from build123d import *

# Parameters (mm, degrees)
F0_W     = 355.6
F0_H     = 355.6
F1_DEPTH = 50.8
F3_DEPTH = 6.35
F4_DEPTH = 6.35


with BuildPart() as f1:
    # F0 (on Front) → F1 (new body)
    with BuildSketch(Plane.XZ):
        Rectangle(F0_W, F0_H)
    extrude(amount=F1_DEPTH)

    # F2 (on face) → F3 (cut)
    with BuildSketch(Plane.XZ.offset(50.8)):
        Polygon((-167.600538, 131.020906), (-171.194881, 122.465245), (101.947516, 55.141423), (104.141387, 64.042271), align=None)
        Polygon((-77.381766, -53.872798), (-73.398896, -66.51783), (163.904211, 8.226743), (162.432873, 21.662845), align=None)
        Polygon((96.553348, -157.102942), (-157.932714, -88.089772), (-160.472856, -99.545852), (93.485428, -168.415896), align=None)
    extrude(amount=-F3_DEPTH, mode=Mode.SUBTRACT)

    # F2 (on face) → F4 (cut)
    with BuildSketch(Plane.XZ.offset(50.8)):
        Polygon((-167.600538, 131.020906), (-171.194881, 122.465245), (101.947516, 55.141423), (104.141387, 64.042271), align=None)
        Polygon((-77.381766, -53.872798), (-73.398896, -66.51783), (163.904211, 8.226743), (162.432873, 21.662845), align=None)
        Polygon((96.553348, -157.102942), (-157.932714, -88.089772), (-160.472856, -99.545852), (93.485428, -168.415896), align=None)
    extrude(amount=-F4_DEPTH, mode=Mode.SUBTRACT)


solid = f1.part
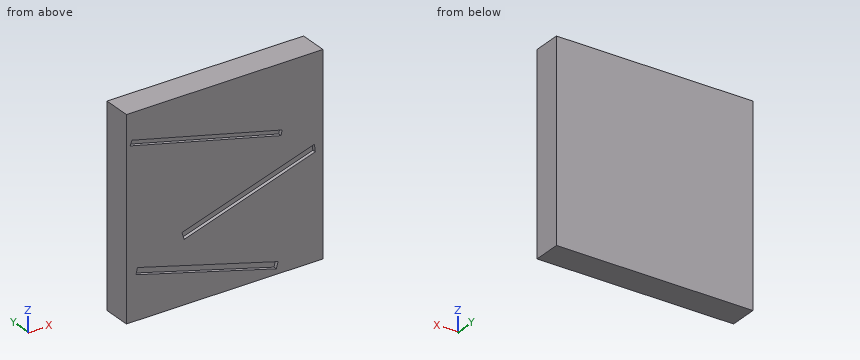
Input: part model. Units: mm. Frame: model coordinates. Give positions to 0.01 mm unless a question says otherwise; leave off trailing zeros. Loops run counter-clockwise (first coordinate to the right, second up) from the corner with the lowest first, then second, coordinate; pieces in that order, holes last. Notation, with made-up numbers: (71, -10) -> (100, -10) arc R28 ccw to (100, 25) -> close; hole circle Ø9 at (-11.75, 27.5). An arc over 180 degrees is marked (long way). Answer as a JSON object with one key per item and string values. Group by question number.
Item 1: Line query: probe 1 along Z at (x, y) = (-153, -45). Output: solid intervals per line, ascending.
Item 2: Cut plane B-B, the plane z = -36.5. Return the cut outline in (x, y), and give its area (3 significant figures).
Item 3: Cut plane A-A, the plane z = -145. Return the cut outline in (x, y), and give its area (3 significant figures).
Checks:
{
 "1": {"probe 1": "z = -177.8 to -101.57, -89.43 to 117.98, 127.42 to 177.8"},
 "2": {"outline": "(-177.8, -50.8) -> (-22.23, -50.8) -> (-22.23, -44.45) -> (21.9, -44.45) -> (21.9, -50.8) -> (177.8, -50.8) -> (177.8, 0) -> (-177.8, 0) -> close", "area": "17,800 mm²"},
 "3": {"outline": "(-177.8, -50.8) -> (7.14, -50.8) -> (7.14, -44.45) -> (51.92, -44.45) -> (51.92, -50.8) -> (177.8, -50.8) -> (177.8, 0) -> (-177.8, 0) -> close", "area": "17,800 mm²"}
}
